Source: CAD feature listing. Evaluate the final solid. Frame: model axes, mm. Round coordinates to 2 decimals unless told otherwise and drop trailing zeros. Use a Markdown table: item, result. Add a question column.
```python
from build123d import *

# Parameters (mm, degrees)
MODEL_R         = 2.15
MODEL_R_2       = 2
EXTRUDE_1_DEPTH = 410


with BuildPart() as part:
    # Model → 보스-돌출1 (new body)
    with BuildSketch(Plane.XY):
        with BuildLine():
            Line((2307.763927197, 1192.134297913), (2307.763927197, 1195.391548465))
            ThreePointArc((2307.763927197, 1195.391548465), (2307.676059232, 1195.603680499), (2307.463927197, 1195.691548465))
            Line((2307.463927197, 1195.691548465), (2306.563927197, 1195.691548465))
            ThreePointArc((2306.563927197, 1195.691548465), (2306.351795163, 1195.779416431), (2306.263927197, 1195.991548465))
            Line((2306.263927197, 1195.991548465), (2306.263927197, 1196.891548465))
            ThreePointArc((2306.263927197, 1196.891548465), (2306.351795163, 1197.103680499), (2306.563927197, 1197.191548465))
            Line((2306.563927197, 1197.191548465), (2313.313927197, 1197.191548465))
            ThreePointArc((2313.313927197, 1197.191548465), (2313.526059232, 1197.103680499), (2313.613927197, 1196.891548465))
            Line((2313.613927197, 1196.891548465), (2313.613927197, 1190.141548465))
            ThreePointArc((2313.613927197, 1190.141548465), (2313.526059232, 1189.929416431), (2313.313927197, 1189.841548465))
            Line((2313.313927197, 1189.841548465), (2312.413927197, 1189.841548465))
            ThreePointArc((2312.413927197, 1189.841548465), (2312.201795163, 1189.929416431), (2312.113927197, 1190.141548465))
            Line((2312.113927197, 1190.141548465), (2312.113927197, 1191.041548465))
            ThreePointArc((2312.113927197, 1191.041548465), (2312.026059232, 1191.253680499), (2311.813927197, 1191.341548465))
            Line((2311.813927197, 1191.341548465), (2308.556676645, 1191.341548465))
            ThreePointArc((2308.556676645, 1191.341548465), (2308.426234796, 1191.311705686), (2308.321744595, 1191.228114625))
            ThreePointArc((2308.321744595, 1191.228114625), (2307.328306374, 1189.47356999), (2306.921204563, 1187.498825831))
            Line((2306.921204563, 1187.498825831), (2306.613927197, 1187.191548465))
            Line((2306.613927197, 1187.191548465), (2306.921204563, 1186.884271099))
            ThreePointArc((2306.921204563, 1186.884271099), (2307.328306374, 1184.90952694), (2308.321744595, 1183.154982305))
            ThreePointArc((2308.321744595, 1183.154982305), (2308.426234796, 1183.071391244), (2308.556676645, 1183.041548465))
            Line((2308.556676645, 1183.041548465), (2311.813927197, 1183.041548465))
            ThreePointArc((2311.813927197, 1183.041548465), (2312.026059232, 1183.129416431), (2312.113927197, 1183.341548465))
            Line((2312.113927197, 1183.341548465), (2312.113927197, 1184.241548465))
            ThreePointArc((2312.113927197, 1184.241548465), (2312.201795163, 1184.453680499), (2312.413927197, 1184.541548465))
            Line((2312.413927197, 1184.541548465), (2313.313927197, 1184.541548465))
            ThreePointArc((2313.313927197, 1184.541548465), (2313.526059232, 1184.453680499), (2313.613927197, 1184.241548465))
            Line((2313.613927197, 1184.241548465), (2313.613927197, 1177.491548465))
            ThreePointArc((2313.613927197, 1177.491548465), (2313.526059232, 1177.279416431), (2313.313927197, 1177.191548465))
            Line((2313.313927197, 1177.191548465), (2306.563927197, 1177.191548465))
            ThreePointArc((2306.563927197, 1177.191548465), (2306.351795163, 1177.279416431), (2306.263927197, 1177.491548465))
            Line((2306.263927197, 1177.491548465), (2306.263927197, 1178.391548465))
            ThreePointArc((2306.263927197, 1178.391548465), (2306.351795163, 1178.603680499), (2306.563927197, 1178.691548465))
            Line((2306.563927197, 1178.691548465), (2307.463927197, 1178.691548465))
            ThreePointArc((2307.463927197, 1178.691548465), (2307.676059232, 1178.779416431), (2307.763927197, 1178.991548465))
            Line((2307.763927197, 1178.991548465), (2307.763927197, 1182.248799017))
            ThreePointArc((2307.763927197, 1182.248799017), (2307.734084418, 1182.379240866), (2307.650493357, 1182.483731067))
            ThreePointArc((2307.650493357, 1182.483731067), (2305.895948722, 1183.477169289), (2303.921204563, 1183.884271099))
            Line((2303.921204563, 1183.884271099), (2303.613927197, 1184.191548465))
            Line((2303.613927197, 1184.191548465), (2303.306649831, 1183.884271099))
            ThreePointArc((2303.306649831, 1183.884271099), (2301.331905673, 1183.477169289), (2299.577361038, 1182.483731067))
            ThreePointArc((2299.577361038, 1182.483731067), (2299.493769977, 1182.379240866), (2299.463927197, 1182.248799017))
            Line((2299.463927197, 1182.248799017), (2299.463927197, 1178.991548465))
            ThreePointArc((2299.463927197, 1178.991548465), (2299.551795163, 1178.779416431), (2299.763927197, 1178.691548465))
            Line((2299.763927197, 1178.691548465), (2300.663927197, 1178.691548465))
            ThreePointArc((2300.663927197, 1178.691548465), (2300.876059232, 1178.603680499), (2300.963927197, 1178.391548465))
            Line((2300.963927197, 1178.391548465), (2300.963927197, 1177.491548465))
            ThreePointArc((2300.963927197, 1177.491548465), (2300.876059232, 1177.279416431), (2300.663927197, 1177.191548465))
            Line((2300.663927197, 1177.191548465), (2293.913927197, 1177.191548465))
            ThreePointArc((2293.913927197, 1177.191548465), (2293.701795163, 1177.279416431), (2293.613927197, 1177.491548465))
            Line((2293.613927197, 1177.491548465), (2293.613927197, 1184.241548465))
            ThreePointArc((2293.613927197, 1184.241548465), (2293.701795163, 1184.453680499), (2293.913927197, 1184.541548465))
            Line((2293.913927197, 1184.541548465), (2294.813927197, 1184.541548465))
            ThreePointArc((2294.813927197, 1184.541548465), (2295.026059232, 1184.453680499), (2295.113927197, 1184.241548465))
            Line((2295.113927197, 1184.241548465), (2295.113927197, 1183.341548465))
            ThreePointArc((2295.113927197, 1183.341548465), (2295.201795163, 1183.129416431), (2295.413927197, 1183.041548465))
            Line((2295.413927197, 1183.041548465), (2298.671177749, 1183.041548465))
            ThreePointArc((2298.671177749, 1183.041548465), (2298.801619599, 1183.071391244), (2298.906109799, 1183.154982305))
            ThreePointArc((2298.906109799, 1183.154982305), (2299.899548021, 1184.90952694), (2300.306649831, 1186.884271099))
            Line((2300.306649831, 1186.884271099), (2300.613927197, 1187.191548465))
            Line((2300.613927197, 1187.191548465), (2300.306649831, 1187.498825831))
            ThreePointArc((2300.306649831, 1187.498825831), (2299.899548021, 1189.47356999), (2298.906109799, 1191.228114625))
            ThreePointArc((2298.906109799, 1191.228114625), (2298.801619599, 1191.311705686), (2298.671177749, 1191.341548465))
            Line((2298.671177749, 1191.341548465), (2295.413927197, 1191.341548465))
            ThreePointArc((2295.413927197, 1191.341548465), (2295.201795163, 1191.253680499), (2295.113927197, 1191.041548465))
            Line((2295.113927197, 1191.041548465), (2295.113927197, 1190.141548465))
            ThreePointArc((2295.113927197, 1190.141548465), (2295.026059232, 1189.929416431), (2294.813927197, 1189.841548465))
            Line((2294.813927197, 1189.841548465), (2293.913927197, 1189.841548465))
            ThreePointArc((2293.913927197, 1189.841548465), (2293.701795163, 1189.929416431), (2293.613927197, 1190.141548465))
            Line((2293.613927197, 1190.141548465), (2293.613927197, 1196.891548465))
            ThreePointArc((2293.613927197, 1196.891548465), (2293.701795163, 1197.103680499), (2293.913927197, 1197.191548465))
            Line((2293.913927197, 1197.191548465), (2300.663927197, 1197.191548465))
            ThreePointArc((2300.663927197, 1197.191548465), (2300.876059232, 1197.103680499), (2300.963927197, 1196.891548465))
            Line((2300.963927197, 1196.891548465), (2300.963927197, 1195.991548465))
            ThreePointArc((2300.963927197, 1195.991548465), (2300.876059232, 1195.779416431), (2300.663927197, 1195.691548465))
            Line((2300.663927197, 1195.691548465), (2299.763927197, 1195.691548465))
            ThreePointArc((2299.763927197, 1195.691548465), (2299.551795163, 1195.603680499), (2299.463927197, 1195.391548465))
            Line((2299.463927197, 1195.391548465), (2299.463927197, 1192.134297913))
            ThreePointArc((2299.463927197, 1192.134297913), (2299.493769977, 1192.003856063), (2299.577361038, 1191.899365863))
            ThreePointArc((2299.577361038, 1191.899365863), (2301.331905673, 1190.905927641), (2303.306649831, 1190.498825831))
            Line((2303.306649831, 1190.498825831), (2303.613927197, 1190.191548465))
            Line((2303.613927197, 1190.191548465), (2303.921204563, 1190.498825831))
            ThreePointArc((2303.921204563, 1190.498825831), (2305.895948722, 1190.905927641), (2307.650493357, 1191.899365863))
            ThreePointArc((2307.650493357, 1191.899365863), (2307.734084418, 1192.003856063), (2307.763927197, 1192.134297913))
        make_face()
        with Locations(Location((2303.613927197, 1187.191548465, 0), (0, 0, 180))):
            Circle(MODEL_R, mode=Mode.SUBTRACT)
        with Locations(Location((2296.613927197, 1194.191548465, 0), (0, 0, 180))):
            Circle(MODEL_R_2, mode=Mode.SUBTRACT)
        with Locations(Location((2296.613927197, 1180.191548465, 0), (0, 0, 180))):
            Circle(MODEL_R_2, mode=Mode.SUBTRACT)
        with Locations(Location((2310.613927197, 1194.191548465, 0), (0, 0, 180))):
            Circle(MODEL_R_2, mode=Mode.SUBTRACT)
        with Locations(Location((2310.613927197, 1180.191548465, 0), (0, 0, 180))):
            Circle(MODEL_R_2, mode=Mode.SUBTRACT)
    extrude(amount=EXTRUDE_1_DEPTH)


solid = part.part
```
1) Line query: probe 1 along X at (y, z) = (1194.25, 240); probe 2 along X at (y, z) = (1180.75, 359.5); probe 3 along Y at (x, z) = (2299, 77). Output: solid intervals per line, ascending. Write a range as from..to.
2) Section A-A on z = 292.5. Count the separate pieces of the cut face and the enclosed holes in it, then the cut area to 3 significant figures.
3) First-contact query: pin 1 Ø2 at (x, y) = (2295.5, 1188) entering from -Z; pin 2 Ø2 at (y, z) = (1186, 353) entering from +X; pin 3 Ø1 at (y, z) = (1189.5, 232) entering from -X; pin 4 Ø1 at (y, z) = (1188, 311) entering from +X. Flat tips, straight axial feed; report the tip coordinate or a pass-through.
Conclusion:
| question | item | result |
|---|---|---|
| 1 | probe 1 | x = 2293.61..2294.61, 2298.61..2299.46, 2307.76..2308.61, 2312.61..2313.61 |
| 1 | probe 2 | x = 2293.61..2294.69, 2298.53..2299.46, 2307.76..2308.69, 2312.53..2313.61 |
| 1 | probe 3 | y = 1177.19..1183.28, 1191.11..1197.19 |
| 2 | separate pieces | 1 |
| 2 | enclosed holes | 5 |
| 2 | area | 146 mm^2 |
| 3 | pin 1 | passes through |
| 3 | pin 2 | stops at x = 2307.3 |
| 3 | pin 3 | stops at x = 2293.65 |
| 3 | pin 4 | stops at x = 2307.05 |
